```python
from build123d import *

# Parameters (mm, degrees)
SKETCH1_W           = 12.5
SKETCH1_H           = 180
BOSS_EXTRUDE1_DEPTH = 20
SKETCH2_R           = 5.65
BOSS_EXTRUDE2_DEPTH = 1.5
SKETCH3_R           = 3.99
BOSS_EXTRUDE3_DEPTH = 7
SKETCH4_R           = 5.65
BOSS_EXTRUDE4_DEPTH = 2.25
SKETCH5_R           = 3.99
BOSS_EXTRUDE5_DEPTH = 7.5
BOSS_EXTRUDE6_START = 2.25
SKETCH6_R           = 5.65
BOSS_EXTRUDE6_DEPTH = 2.25
BOSS_EXTRUDE7_START = 7.5
SKETCH7_R           = 3.99
BOSS_EXTRUDE7_DEPTH = 7.5
SKETCH8_R           = 3.95
CUT_EXTRUDE1_DEPTH  = 19
SKETCH9_W           = 8
SKETCH9_H           = 2
CUT_EXTRUDE2_DEPTH  = 72.5
SKETCH10_W          = 11.5
SKETCH10_H          = 1
CUT_EXTRUDE3_DEPTH  = 72.5
CUT_EXTRUDE5_DEPTH  = 20
SKETCH14_W          = 4
SKETCH14_H          = 5
CUT_EXTRUDE6_DEPTH  = 12.5
CUT_EXTRUDE7_REACH  = 104.943


with BuildPart() as part:
    # Sketch1 → Boss-Extrude1 (new body)
    with BuildSketch(Plane(origin=(0, 0, 0), x_dir=(1, 0, 0), z_dir=(0, 1, 0))):
        Rectangle(SKETCH1_W, SKETCH1_H)
    extrude(amount=BOSS_EXTRUDE1_DEPTH)

    # Sketch2 → Boss-Extrude2 (add)
    with BuildSketch(Plane.XY.offset(90)):
        with Locations(Location((0, 10, 0), (0, 0, 180))):
            Circle(SKETCH2_R)
    extrude(amount=BOSS_EXTRUDE2_DEPTH)

    # Sketch3 → Boss-Extrude3 (add)
    with BuildSketch(Plane.XY.offset(91.5)):
        with Locations(Location((0, 10, 0), (0, 0, 180))):
            Circle(SKETCH3_R)
    extrude(amount=BOSS_EXTRUDE3_DEPTH)

    # Sketch4 → Boss-Extrude4 (add)
    with BuildSketch(Plane.ZY.offset(6.25)):
        with Locations(Location((0, 10, 0), (0, 0, 180))):
            Circle(SKETCH4_R)
    extrude(amount=BOSS_EXTRUDE4_DEPTH)

    # Sketch5 → Boss-Extrude5 (add)
    with BuildSketch(Plane.ZY.offset(8.5)):
        with Locations((0, 10)):
            Circle(SKETCH5_R)
    extrude(amount=BOSS_EXTRUDE5_DEPTH)

    # Sketch6 → Boss-Extrude6 (add)
    with BuildSketch(Plane(origin=(6.25, 0, 0), x_dir=(0, 0, -1), z_dir=(1, 0, 0)).offset(BOSS_EXTRUDE6_START)):
        with Locations((0, 10)):
            Circle(SKETCH6_R)
    extrude(amount=-BOSS_EXTRUDE6_DEPTH)

    # Sketch7 → Boss-Extrude7 (add)
    with BuildSketch(Plane(origin=(8.5, 0, 0), x_dir=(0, 0, -1), z_dir=(1, 0, 0)).offset(BOSS_EXTRUDE7_START)):
        with Locations(Location((0, 10, 0), (0, 0, 180))):
            Circle(SKETCH7_R)
    extrude(amount=-BOSS_EXTRUDE7_DEPTH)

    # Sketch8 → Cut-Extrude1 (cut)
    with BuildSketch(Plane(origin=(0, 20, 0), x_dir=(1, 0, 0), z_dir=(0, 1, 0))):
        with Locations(Location((0, 82.5, 0), (0, 0, 270))):
            Circle(SKETCH8_R)
        with Locations(Location((0, 72.5, 0), (0, 0, 270))):
            Circle(SKETCH8_R)
        with Locations(Location((0, 62.5, 0), (0, 0, 270))):
            Circle(SKETCH8_R)
        with Locations(Location((0, 52.5, 0), (0, 0, 270))):
            Circle(SKETCH8_R)
        with Locations(Location((0, 42.5, 0), (0, 0, 270))):
            Circle(SKETCH8_R)
        with Locations(Location((0, 32.5, 0), (0, 0, 270))):
            Circle(SKETCH8_R)
        with Locations(Location((0, 22.5, 0), (0, 0, 270))):
            Circle(SKETCH8_R)
    extrude(amount=-CUT_EXTRUDE1_DEPTH, mode=Mode.SUBTRACT)

    # Sketch9 → Cut-Extrude2 (cut)
    with BuildSketch(Plane(origin=(0, 0, -90), x_dir=(-1, 0, 0), z_dir=(0, 0, -1))):
        with Locations((0, 18)):
            Rectangle(SKETCH9_W, SKETCH9_H)
    extrude(amount=-CUT_EXTRUDE2_DEPTH, mode=Mode.SUBTRACT)

    # Sketch10 → Cut-Extrude3 (cut)
    with BuildSketch(Plane(origin=(0, 0, -90), x_dir=(-1, 0, 0), z_dir=(0, 0, -1))):
        with Locations((0, 18)):
            Rectangle(SKETCH10_W, SKETCH10_H)
    extrude(amount=-CUT_EXTRUDE3_DEPTH, mode=Mode.SUBTRACT)

    # Sketch12 → Cut-Extrude5 (cut)
    with BuildSketch(Plane.XY.offset(98.5)):
        with BuildLine():
            Line((1.936491673, 10.5), (2.5, 10.5))
            Line((2.5, 10.5), (2.5, 9.5))
            Line((2.5, 9.5), (1.936491673, 9.5))
            ThreePointArc((1.936491673, 9.5), (0, 8), (-1.936491673, 9.5))
            Line((-1.936491673, 9.5), (-2.5, 9.5))
            Line((-2.5, 9.5), (-2.5, 10.5))
            Line((-2.5, 10.5), (-1.936491673, 10.5))
            ThreePointArc((-1.936491673, 10.5), (0, 12), (1.936491673, 10.5))
        make_face()
    extrude(amount=-CUT_EXTRUDE5_DEPTH, mode=Mode.SUBTRACT)

    # Sketch14 → Cut-Extrude6 (cut)
    with BuildSketch(Plane(origin=(6.25, 0, 0), x_dir=(0, 0, -1), z_dir=(1, 0, 0))):
        with Locations((-15, 10)):
            Rectangle(SKETCH14_W, SKETCH14_H)
    extrude(amount=-CUT_EXTRUDE6_DEPTH, mode=Mode.SUBTRACT)

    # Sketch15 → Cut-Extrude7 (cut, up to next)
    with BuildSketch(Plane(origin=(6.25, 0, 0), x_dir=(0, 0, -1), z_dir=(1, 0, 0)), mode=Mode.PRIVATE) as cut_extrude7_sk1:
        Polygon((-60, 10), (-60, 20), (-22.30384635, 20), align=None)
    cut_extrude7_tool1 = extrude(cut_extrude7_sk1.sketch, amount=-CUT_EXTRUDE7_REACH, mode=Mode.PRIVATE) & part.part
    add(cut_extrude7_tool1.solids().sort_by_distance((6.25, 16.666667, 47.434615))[0], mode=Mode.SUBTRACT)


solid = part.part
```
CAD build for the part. Positions are in the model's coordinates, mm. A direction names the side the tool comes from. Round coordinates to 2 decimals unless told otherwise and drop trailing zeros. Loops run counter-clockwise (first coordinate to the right, second up) from the corner with the lowest first, then second, coordinate; pieces in that order, holes last. Notation, with made-up numbers: (-6.5, -31.75) - (21.5, -31.75) arc R23 ccw to (21.5, 0.25) - close; hole circle Ø4 at (-19, 22.25). An arc over 180 degrees is marked (long way). Return JSON: item names as keys, results as strings. Group by question number.
Q1. Band-saw the part on A-A on x = 0. Give the number of separate pieces and of enclosed holes in the cut face, plus the area to 3 significant figures.
Q2. Band-saw the part on C-C on z = -32.5. Give the cut face in (x, y), plus the area to 3 significant figures.
Q3. Band-saw the part on B-B on y = 2.75. Give the cut face in (x, z), plus the area to 3 significant figures.
Q4. Band-saw the part on D-D on x = 13.5. Give the cut face in (y, z).
Q5. Drill centre lines: line 1 along X through (y, z) = (19.6, -52.5); line 2 along Y through (x, z) = (5.5, -70.5); line 3 along Y through (x, z) = (2, -27). Where is each one in solid material? Low to high. Write a range as [from, to].
Q6. Flat gauge pins, fed straight in: pin 1 Ø2 at (x, z) = (-2.5, 48.5) entering from +Y; pin 2 Ø4.5 at (x, z) = (0, -32.5) entering from +Y; pin 3 Ø1.5 at (x, y) = (-1, 9.5) entering from +Z. Where does each tip first touch, or does it go through?
Q7. Two-plate mould, pull along X, no slides. Class faces 1 (the face through (0, 15, 60)), 2 (the face through (0.174, 19.507, -86.446)), 3 (the face through (-16, 10, 0)): +X half, -X half, draft (parallel to the pull), parting line (faces both ways), or undercut.
Q8. Tool access for faces 4 (the face through (0, 12, 89)), 5 (the face through (0, 1, -43)), 6 (the face through (3.6, 17, -70.4)), 7 (the face through (0, 10, 17)), 8 (the face through (7.39, 15.6, 0.74)): list every direction of +Z, -Z, +X, -X, +Y, -Y with a clear straight run to the whole face (end or side of a thin tool).
Solutions:
{
 "1": {"separate pieces": "8", "enclosed holes": "1", "area": "2,300 mm^2"},
 "2": {"outline": "(-6.25, 0) - (6.25, 0) - (6.25, 20) - (3.95, 20) - (3.95, 19) - (4, 19) - (4, 18.5) - (5.75, 18.5) - (5.75, 17.5) - (4, 17.5) - (4, 17) - (3.95, 17) - (3.95, 1) - (-3.95, 1) - (-3.95, 17) - (-4, 17) - (-4, 17.5) - (-5.75, 17.5) - (-5.75, 18.5) - (-4, 18.5) - (-4, 19) - (-3.95, 19) - (-3.95, 20) - (-6.25, 20) - close", "area": "96.2 mm^2"},
 "3": {"outline": "(-6.25, -90) - (6.25, -90) - (6.25, 90) - (-6.25, 90) - close; hole circle Ø7.9 at (0, -82.5); hole circle Ø7.9 at (0, -72.5); hole circle Ø7.9 at (0, -62.5); hole circle Ø7.9 at (0, -52.5); hole circle Ø7.9 at (0, -42.5); hole circle Ø7.9 at (0, -32.5); hole circle Ø7.9 at (0, -22.5)", "area": "1,910 mm^2"},
 "4": {"outline": "circle Ø7.98 at (10, 0)"},
 "5": {"line 1": "x = [-6.25, -3.95], [3.95, 6.25]", "line 2": "y = [0, 17.5], [18.5, 20]", "line 3": "y = [0, 17], [19, 20]"},
 "6": {"pin 1": "stops at y = 13.32", "pin 2": "stops at y = 1", "pin 3": "stops at z = 78.5"},
 "7": {"face 1": "draft", "face 2": "undercut", "face 3": "-X half"},
 "8": {"face 4": "+Z", "face 5": "+Y", "face 6": "-Z", "face 7": "+X, -X", "face 8": "+X"}
}
